```python
from build123d import *

# Parameters (mm, degrees)
SKIZZE1_R                            = 8
AUFSATZ_LINEAR_AUSTRAGEN1_DEPTH      = 26
SKIZZE2_R                            = 6.5
AUFSATZ_LINEAR_AUSTRAGEN2_DEPTH      = 3
SCHNITT_LINEAR_AUSTRAGEN1_DEPTH      = 32.128764833
SCHNITT_LINEAR_AUSTRAGEN1_DEPTH_BACK = 32.128764833
SKIZZE3_R                            = 5
FASE1_SIZE                           = 0.2


with BuildPart() as part:
    # Skizze1 → Aufsatz-Linear austragen1 (new body)
    with BuildSketch(Plane.XY):
        with Locations(Location((0, 0, 0), (0, 0, 180))):
            Circle(SKIZZE1_R)
    extrude(amount=AUFSATZ_LINEAR_AUSTRAGEN1_DEPTH)

    # Skizze2 → Aufsatz-Linear austragen2 (add)
    with BuildSketch(Plane.XY.offset(26)):
        Circle(SKIZZE2_R)
    extrude(amount=AUFSATZ_LINEAR_AUSTRAGEN2_DEPTH)

    # Skizze3 → Schnitt-Linear austragen1 (cut, two sides: drawn at the far end of the back side and taken through both)
    with BuildSketch(Plane(origin=(0, 0, 0), x_dir=(-1, 0, 0), z_dir=(0, 0, -1)).offset(-SCHNITT_LINEAR_AUSTRAGEN1_DEPTH_BACK)):
        Circle(SKIZZE3_R)
    extrude(amount=SCHNITT_LINEAR_AUSTRAGEN1_DEPTH + SCHNITT_LINEAR_AUSTRAGEN1_DEPTH_BACK, mode=Mode.SUBTRACT)

    # Fase1
    fase1_edges = [part.edges().sort_by_distance(p)[0] for p in [
        (8, 0, 0),
        (8, 0, 26),
        (-6.5, 0, 29),
    ]]
    chamfer(fase1_edges, length=FASE1_SIZE)


solid = part.part
```
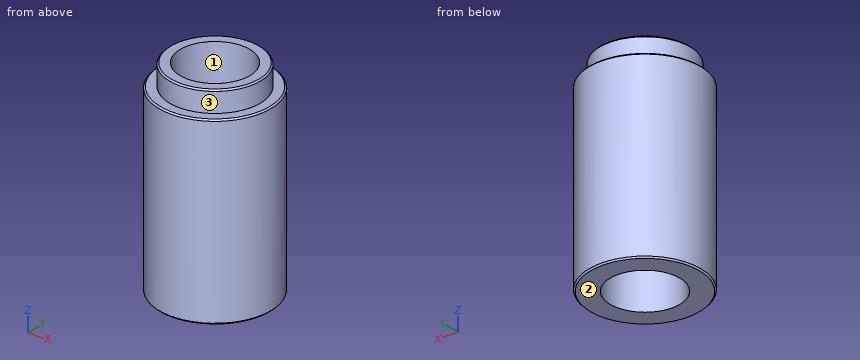
Input: part model. Units: mm. Frame: model coordinates. Face numbers are marked on the shaded views. Coordinates: 2 decimals unless noted, no trailing zeros. Write each loop counter-clockwise with the first axis right and the second up, starting at its lowest first coordinate (ties: lowest second). Pieces come first, ordered by that corner, then holes.
1) Mould query, pull axis X, two halves, no side actions, for the marked faces 1, 2 and 3. Classes: pulls with the +X half, pulls with the -X half, needs draft (parallel to the pull), parting line crosses it, or undercut.
2) Section A-A on x = 0. Output: boundary loops of the cut face in (y, z).
3) Pin query (flat end, axial travel): pin 1 Ø1 at (y, z) = (-5, 12) entering from +X. Return the tip coordinate at first contact, or that it passes through.
4) Section C-C on z = 4.5. Output: boundary loops of the cut face in (x, y), and give its area (3 significant figures).
5) Material intervals for line 1 along Y through (x, z) = (0, 7.5); line 2 along Z through (x, y) = (-4.5, -6); line 3 along X through (y, z) = (1.75, 19.75), sorted ascending.
Check result:
1. face 1: undercut
1. face 2: needs draft
1. face 3: parting line crosses it
2. outline: (-8, 0.2) - (-7.8, 0) - (-5, 0) - (-5, 29) - (-6.3, 29) - (-6.5, 28.8) - (-6.5, 26) - (-7.8, 26) - (-8, 25.8) - close; (5, 0) - (7.8, 0) - (8, 0.2) - (8, 25.8) - (7.8, 26) - (6.5, 26) - (6.5, 28.8) - (6.3, 29) - (5, 29) - close
3. pin 1: stops at x = 6.61
4. outline: circle Ø16 at (0, 0); hole circle Ø10 at (0, 0)
4. area: 123 mm2
5. line 1: y = -8 to -5, 5 to 8
5. line 2: z = 0 to 26
5. line 3: x = -7.81 to -4.68, 4.68 to 7.81
